from build123d import *

# Parameters (mm, degrees)
SKETCH_1_W          = 105
SKETCH_1_H          = 90
EXTRUDE_1_DEPTH     = 25
SHELL_1_T           = -2
SKETCH_8_R          = 2.15
EXTRUDE_3_DEPTH     = 5
SKETCH_3_W          = 24
SKETCH_3_H          = 7.5
SKETCH_3_W_2        = 14.9
CUT_EXTRUDE_2_DEPTH = 10
SKETCH_5_W          = 24.5
SKETCH_5_H          = 7.5
CUT_EXTRUDE_3_DEPTH = 10
SKETCH_7_W          = 33.5
SKETCH_7_H          = 7.5
SKETCH_7_W_2        = 16.5
SKETCH_7_W_3        = 24
CUT_EXTRUDE_4_DEPTH = 10
SKETCH_9_R          = 1.5
CUT_EXTRUDE_5_DEPTH = 50
SKETCH_2_R          = 1.4
SKETCH_2_W          = 9
SKETCH_2_H          = 10
EXTRUDE_6_DEPTH     = 6
SKETCH_3_8_W        = 24
SKETCH_3_8_H        = 7.5
SKETCH_3_8_W_2      = 14.9
SKETCH_3_8_W_3      = 13
SKETCH_3_8_H_2      = 10
CUT_EXTRUDE_6_DEPTH = 10


with BuildPart() as part:
    # Sketch 1 → Extrude 1 (new body)
    with BuildSketch(Plane(origin=(0, 0, 0), x_dir=(1, 0, 0), z_dir=(0, 1, 0))):
        Rectangle(SKETCH_1_W, SKETCH_1_H)
    extrude(amount=EXTRUDE_1_DEPTH)

    # Shell 1
    shell_1_openings = [part.faces().sort_by_distance(p)[0] for p in [
        (0, 25, 0),
    ]]
    offset(amount=SHELL_1_T, openings=shell_1_openings, kind=Kind.INTERSECTION)

    # Sketch 8 → Extrude 3 (add)
    with BuildSketch(Plane.XZ):
        with BuildLine():
            Line((-57.5, 5), (-52.5, 5))
            Line((-52.5, 5), (-52.5, -5))
            Line((-52.5, -5), (-57.5, -5))
            ThreePointArc((-57.5, -5), (-62.5, 0), (-57.5, 5))
        make_face()
        with Locations((-57.5, 0)):
            Circle(SKETCH_8_R, mode=Mode.SUBTRACT)
        with BuildLine():
            Line((52.5, -5), (57.5, -5))
            ThreePointArc((57.5, -5), (62.5, 0), (57.5, 5))
            Line((57.5, 5), (52.5, 5))
            Line((52.5, 5), (52.5, -5))
        make_face()
        with Locations((57.5, 0)):
            Circle(SKETCH_8_R, mode=Mode.SUBTRACT)
    extrude(amount=-EXTRUDE_3_DEPTH)

    # Sketch 3 → Cut-Extrude 2 (cut)
    with BuildSketch(Plane.XY.offset(45)):
        with Locations((28, 13.55)):
            Rectangle(SKETCH_3_W, SKETCH_3_H)
        with Locations((-11.55, 13.55)):
            Rectangle(SKETCH_3_W_2, SKETCH_3_H)
    extrude(amount=-CUT_EXTRUDE_2_DEPTH, mode=Mode.SUBTRACT)

    # Sketch 5 → Cut-Extrude 3 (cut)
    with BuildSketch(Plane(origin=(52.5, 0, 0), x_dir=(0, 0, -1), z_dir=(1, 0, 0))):
        with Locations((16.55, 13.55)):
            Rectangle(SKETCH_5_W, SKETCH_5_H)
        with Locations((-13.5, 13.471843212)):
            Rectangle(SKETCH_5_W, SKETCH_5_H)
    extrude(amount=-CUT_EXTRUDE_3_DEPTH, mode=Mode.SUBTRACT)

    # Sketch 7 → Cut-Extrude 4 (cut)
    with BuildSketch(Plane(origin=(0, 0, -45), x_dir=(-1, 0, 0), z_dir=(0, 0, -1))):
        with Locations((22.55, 13.55)):
            Rectangle(SKETCH_7_W, SKETCH_7_H)
        with Locations((-5.85, 13.55)):
            Rectangle(SKETCH_7_W_2, SKETCH_7_H)
        with Locations((-28, 13.452632976)):
            Rectangle(SKETCH_7_W_3, SKETCH_7_H)
    extrude(amount=-CUT_EXTRUDE_4_DEPTH, mode=Mode.SUBTRACT)

    # Sketch 9 → Cut-Extrude 5 (cut)
    with BuildSketch(Plane.XY):
        with Locations((0, 18)):
            Circle(SKETCH_9_R)
    extrude(amount=CUT_EXTRUDE_5_DEPTH, mode=Mode.SUBTRACT)

    # Sketch 2 → Extrude 6 (add)
    with BuildSketch(Plane(origin=(0, 2, 0), x_dir=(1, 0, 0), z_dir=(0, 1, 0))):
        Polygon((-41.5, 33), (-41.5, 39), (9.5, 39), (9.5, 43), (-41.5, 43), (-50.5, 43), (-50.5, 33), align=None)
        with Locations((-46.689481309, 39.196373095)):
            Circle(SKETCH_2_R, mode=Mode.SUBTRACT)
        with BuildLine():
            Line((45.5, 43), (38, 43))
            Line((38, 43), (38, 33))
            Line((38, 33), (45.5, 33))
            Line((45.5, 33), (45.5, -32.46))
            ThreePointArc((45.5, -32.46), (45.048944443, -33.548944443), (43.96, -34))
            Line((43.96, -34), (42.04, -34))
            ThreePointArc((42.04, -34), (40.951055557, -34.451055557), (40.5, -35.54))
            Line((40.5, -35.54), (40.5, -43))
            Line((40.5, -43), (50.5, -43))
            Line((50.5, -43), (50.5, 43))
            Line((50.5, 43), (45.5, 43))
        make_face()
        with Locations((46.687886977, -39.208970538)):
            Circle(SKETCH_2_R, mode=Mode.SUBTRACT)
        with Locations((46.691741848, 39.161577941)):
            Circle(SKETCH_2_R, mode=Mode.SUBTRACT)
        with Locations((-46, -38)):
            Rectangle(SKETCH_2_W, SKETCH_2_H)
        with Locations((-46.725108279, -39.220894808)):
            Circle(SKETCH_2_R, mode=Mode.SUBTRACT)
    extrude(amount=EXTRUDE_6_DEPTH)

    # Sketch 3_8 → Cut-Extrude 6 (cut)
    with BuildSketch(Plane.XY.offset(45)):
        with Locations((28, 13.55)):
            Rectangle(SKETCH_3_8_W, SKETCH_3_8_H)
        with Locations((-11.55, 13.55)):
            Rectangle(SKETCH_3_8_W_2, SKETCH_3_8_H)
        with Locations((-31.5, 12.3)):
            Rectangle(SKETCH_3_8_W_3, SKETCH_3_8_H_2)
    extrude(amount=-CUT_EXTRUDE_6_DEPTH, mode=Mode.SUBTRACT)


solid = part.part
Source: CAD feature listing. Evaluate the final solid. Frame: model axes, mm. A direction names the side the tool comes from. Round coordinates to 2 decimals unless told otherwise and drop trailing zeros. Loops run counter-clockwise (first coordinate to the right, second up) from the corner with the lowest first, then second, coordinate; pieces in that order, holes last.
Q1. First-contact query: P1, Ø1.2, axis at y = 5, z = -41.5, coming from the +X side; P2, Ø10, axis at x = -28, z = -30, coming from the +Y side; P3, Ø1.6, axis at y = 15, z = 44, coming from the -X side. Flat tips, straight axial feed; report the tip coordinate or a pass-through.
Q2. Ray query, line 1 (Z direction, x = -45, y = 21.5); line 2 (X direction, y = 14.75, z = 29.5); line 3 (X direction, y = 7.25, z = 18). Return the intervals inside material, ascending.
Q3. Section A-A, the plane z = -11.5. Return loops of the section in (x, y), plus the area to 3 significant figures.
Q4. Section B-B, the plane x = 0. Return loops of the section in (y, z), plus the area to 3 significant figures.
Q5. Section C-C, the plane z = 0. Return loops of the section in (x, y).
Q6. Access query for faces 1 (the face through (-55, 2, -5)), 2 (the face through (-0.195, 19.487, 43.986)), 3 (the face through (-59.65, 2.46, 0.09)), 4 (the face through (47, 8, -1)). Directions: +Z, -Z, +X, -X, +Y, -Y. A direction counts if a zero-diameter tool reaches every point of the face in a straight line with its end or side. Return the directions, or none.
Q7. Section D-D, the plane y = 12.75. State how many separate pieces and enclosed holes the cut face has, plus the area to 3 significant figures.
Q8. Mould query, pull axis Z, two halves, no side actions, for faces 5 (the face through (-51, 25, 0)), 6 (the face through (50.5, 16, 1)), 7 (the face through (-0.7, 9.5, -45)). Classes: pulls with the +Z half, pulls with the -Z half, needs draft (parallel to the pull), parting line crosses it, or undercut.
Solutions:
1. P1: stops at x = 52.5
1. P2: stops at y = 2
1. P3: stops at x = -52.5
2. line 1: z = -45 to -43, 43 to 45
2. line 2: x = -52.5 to -50.5, 50.5 to 52.5
2. line 3: x = -52.5 to -50.5, 45.5 to 52.5
3. outline: (-52.5, 0) - (52.5, 0) - (52.5, 9.8) - (50.5, 9.8) - (50.5, 8) - (45.5, 8) - (45.5, 2) - (-50.5, 2) - (-50.5, 25) - (-52.5, 25) - close; (50.5, 17.3) - (52.5, 17.3) - (52.5, 25) - (50.5, 25) - close
3. area: 317 mm2
4. outline: (0, -45) - (9.8, -45) - (9.8, -43) - (8, -43) - (8, -39) - (2, -39) - (2, 43) - (16.5, 43) - (16.5, 45) - (0, 45) - close; (17.3, -45) - (25, -45) - (25, -43) - (17.3, -43) - close; (19.5, 43) - (25, 43) - (25, 45) - (19.5, 45) - close
4. area: 275 mm2
5. outline: (-62.5, 0) - (-59.65, 0) - (-59.65, 5) - (-62.5, 5) - close; (-55.35, 0) - (55.35, 0) - (55.35, 5) - (52.5, 5) - (52.5, 25) - (50.5, 25) - (50.5, 8) - (45.5, 8) - (45.5, 2) - (-50.5, 2) - (-50.5, 25) - (-52.5, 25) - (-52.5, 5) - (-55.35, 5) - close; (59.65, 0) - (62.5, 0) - (62.5, 5) - (59.65, 5) - close
6. face 1: -Z, -X, +Y, -Y
6. face 2: +Z
6. face 3: +Y, -Y
6. face 4: +Y
7. separate pieces: 8
7. enclosed holes: 0
7. area: 414 mm2
8. face 5: needs draft
8. face 6: undercut
8. face 7: pulls with the -Z half
